Part print with two shaded views. Sizes in mm from the minimum x, y, z corner. A direction names the side the tool comes from. Give positions to 0.01 mm unless a question says otherwise; leave off trailing zeros. Write each loop counter-clockwise with the first axis right and the second up, starting at its lowest first coordinate (ties: lowest second). Pieces come first, ordered by that corner, then holes.
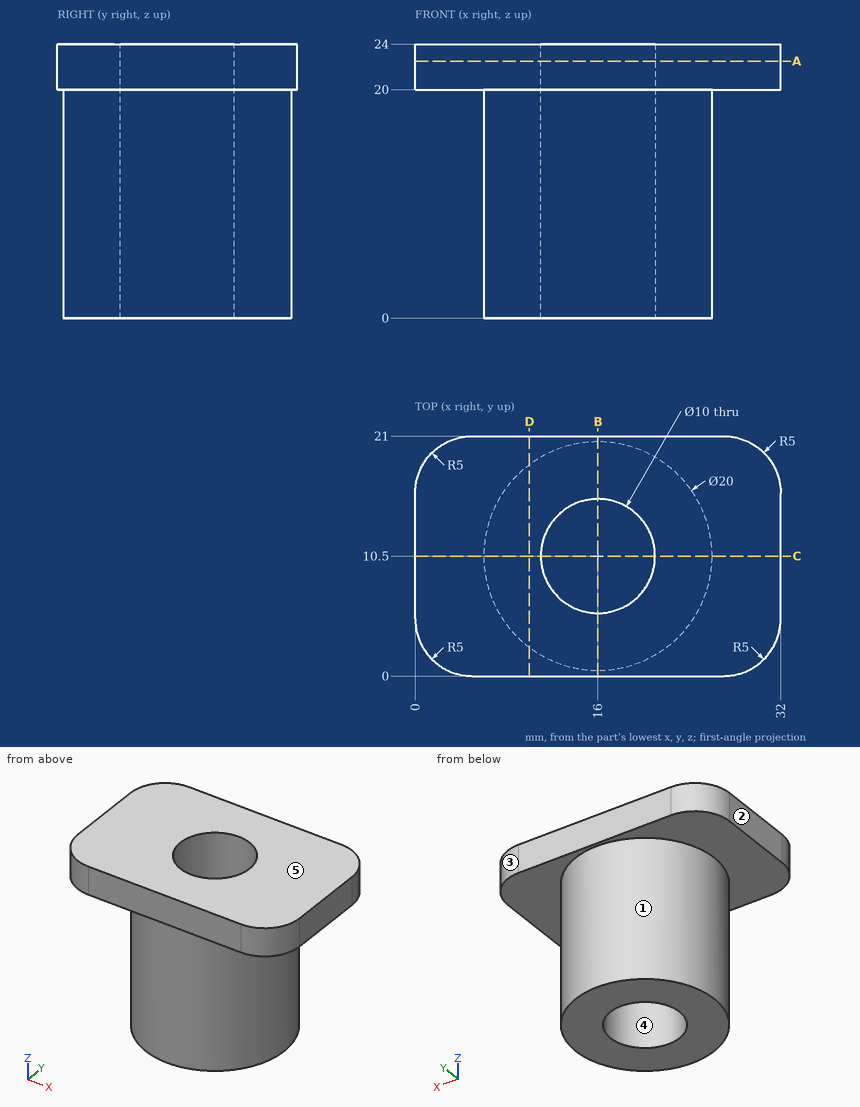
1) Wall check: L1, parallel to Y at x = 16, z = 12; L2, parallel to Z at x = 26, y = 19.75; L3, parallel to X at y = 10.75, z = 14. Give the ranges that are in metal, low to high.
Answers follow:
L1: y = 0.5 to 5.5, 15.5 to 20.5
L2: z = 20 to 24
L3: x = 6 to 11.01, 20.99 to 26
2) Two-plate mould, pull along X, no slides. Class the marked faces 3, 4 and 5: +X half, -X half, draft (parallel to the pull), parting line (faces both ways), or undercut.
Answers follow:
face 3: +X half
face 4: undercut
face 5: draft
3) Saw through at D-D, the plane x = 10. Write the cut outline in (y, z), then the cut area to 3 significant figures.
Answers follow:
outline: (0, 20) - (2.5, 20) - (2.5, 0) - (18.5, 0) - (18.5, 20) - (21, 20) - (21, 24) - (0, 24) - close
area: 404 mm2
4) Saw through at A-A, the plane z = 22.5. Write the cut outline in (x, y).
Answers follow:
outline: (0, 5) arc R5 ccw to (5, 0) - (27, 0) arc R5 ccw to (32, 5) - (32, 16) arc R5 ccw to (27, 21) - (5, 21) arc R5 ccw to (0, 16) - close; hole circle Ø10 at (16, 10.5)
5) Saw through at B-B, the plane x = 16. Write the cut outline in (y, z).
Answers follow:
outline: (0, 20) - (0.5, 20) - (0.5, 0) - (5.5, 0) - (5.5, 24) - (0, 24) - close; (15.5, 0) - (20.5, 0) - (20.5, 20) - (21, 20) - (21, 24) - (15.5, 24) - close
6) Pin check, flat tips, straight feed: pin 1 Ø2 at (x, y) = (26.5, 17.5) entering from -Z; pin 2 Ø6 at (y, z) = (6.5, 9) entering from +X; pin 3 Ø5 at (y, z) = (3.5, 8) entering from -X. Stop position of each tip, or through.
Answers follow:
pin 1: stops at z = 20
pin 2: stops at x = 25.95
pin 3: stops at x = 7.07
7) Saw through at C-C, the plane y = 10.5. Write the cut outline in (x, z).
Answers follow:
outline: (0, 20) - (6, 20) - (6, 0) - (11, 0) - (11, 24) - (0, 24) - close; (21, 0) - (26, 0) - (26, 20) - (32, 20) - (32, 24) - (21, 24) - close
8) 3-axis set-ups, long thin cutter, end or side, ignore diameter. For the marked faces 1 and 2: which of +Z, -Z, +X, -X, +Y, -Y reach the whole face in a straight line?
Answers follow:
face 1: -Z
face 2: +Z, -Z, -X, +Y, -Y
